Model file for the job. Use its own axes, mm. Face numbers are marked on the shaded views. Coordinates: 2 decimals unless noted, no trailing zeros. Order: outer loops, then holes, each group sorted by start corner. A loop starts at its lowest first (then second) coordinate and runs counter-clockwise, first axis right, second up.
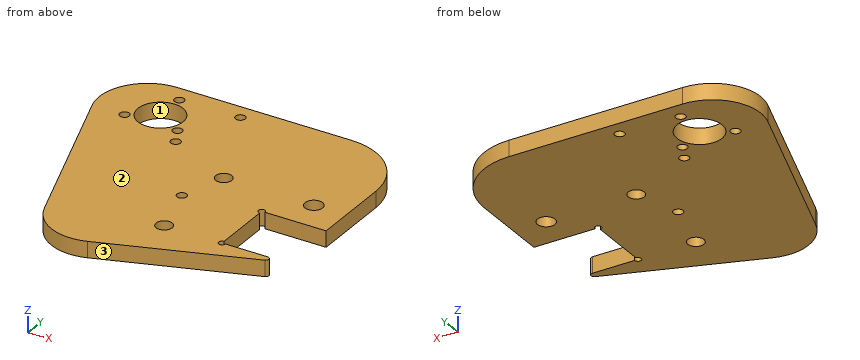
from build123d import *

# Parameters (mm, degrees)
SKETCH_1_R          = 7
SKETCH_1_R_2        = 1.5
SKETCH_1_R_3        = 2.5
EXTRUDE_1_DEPTH     = 5
FILLET_1_R          = 1
SKETCH_2_R          = 1.5
SKETCH_2_R_2        = 2.75
CUT_EXTRUDE_1_DEPTH = 10
SKETCH_3_R          = 1.5
CUT_EXTRUDE_2_DEPTH = 10
SKETCH_4_R          = 1.025
CUT_EXTRUDE_3_DEPTH = 30


with BuildPart() as part:
    # 草图1 → 凸台-拉伸1 (new body)
    with BuildSketch(Plane.XY):
        with BuildLine():
            Line((70, -30), (70, -5))
            ThreePointArc((70, -5), (64.142135624, 9.142135624), (50, 15))
            Line((50, 15), (-4.038673683, 15))
            ThreePointArc((-4.038673683, 15), (-16.237067712, 8.729214347), (-18.236326506, -4.840108917))
            Line((-18.236326506, -4.840108917), (0.10369211, -58.637496855))
            ThreePointArc((0.10369211, -58.637496855), (7.762372735, -67.297085809), (19.305024689, -67.938222033))
            Line((19.305024689, -67.938222033), (70, -50))
            Line((70, -50), (50, -50))
            Line((50, -50), (50, -30))
            Line((50, -30), (70, -30))
        make_face()
        Circle(SKETCH_1_R, mode=Mode.SUBTRACT)
        with Locations((0, 9.5)):
            Circle(SKETCH_1_R_2, mode=Mode.SUBTRACT)
        with Locations((8.227241336, -4.75)):
            Circle(SKETCH_1_R_2, mode=Mode.SUBTRACT)
        with Locations((-8.227241336, -4.75)):
            Circle(SKETCH_1_R_2, mode=Mode.SUBTRACT)
        with Locations((32, -50)):
            Circle(SKETCH_1_R_3, mode=Mode.SUBTRACT)
        with Locations((32, -20)):
            Circle(SKETCH_1_R_3, mode=Mode.SUBTRACT)
    extrude(amount=EXTRUDE_1_DEPTH)

    # 圆角1
    fillet_1_edges = [part.edges().sort_by_distance(p)[0] for p in [
        (70, -50, 2.5),
    ]]
    fillet(fillet_1_edges, radius=FILLET_1_R)

    # 草图2 → 切除-拉伸1 (cut)
    with BuildSketch(Plane.XY.offset(5)):
        with Locations((27.5, -33.82)):
            Circle(SKETCH_2_R)
        with Locations((18.66, 10)):
            Circle(SKETCH_2_R)
        with Locations((60, -20)):
            Circle(SKETCH_2_R_2)
    extrude(amount=-CUT_EXTRUDE_1_DEPTH, mode=Mode.SUBTRACT)

    # 草图3 → 切除-拉伸2 (cut)
    with BuildSketch(Plane.XY.offset(5)):
        with Locations((10.914424012, -10)):
            Circle(SKETCH_3_R)
    extrude(amount=-CUT_EXTRUDE_2_DEPTH, mode=Mode.SUBTRACT)

    # 草图4 → 切除-拉伸3 (cut, symmetric)
    with BuildSketch(Plane(origin=(0, 0, 0), x_dir=(-1, 0, 0), z_dir=(0, 0, -1))):
        with Locations((-50, -50)):
            Circle(SKETCH_4_R)
        with Locations((-50, -30)):
            Circle(SKETCH_4_R)
    extrude(amount=CUT_EXTRUDE_3_DEPTH, both=True, mode=Mode.SUBTRACT)


solid = part.part
Q1. Cut at A-A, the plane z = 1. Count the separate pieces of the cut face and the enclosed holes in it, plus the area to 3 significant figures.
Established:
separate pieces: 1
enclosed holes: 10
area: 5,390 mm2
Q2. Probe line 1 (Y direction, x = 1, z = 4); line 2 (X direction, y = -22, z = 0.4); line 3 (Y direction, x = 32, z = 1.95). List the from-to ranges inside material, lowest first.
Established:
line 1: y = -60.73 to -6.93, 6.93 to 8.38, 10.62 to 15
line 2: x = -12.39 to 30.5, 33.5 to 58.11, 61.89 to 70
line 3: y = -63.45 to -52.5, -47.5 to -22.5, -17.5 to 15
Q3. Cut at D-D, the plane y = -56. List the corners of the cut face in (x, z), plus the area to 3 significant figures.
Established:
outline: (-0.8, 0) - (53.04, 0) - (53.04, 5) - (-0.8, 5) - close
area: 269 mm2
Q4. Cut at C-C, the plane x = 5. List the corners of the cut face in (y, z), plus the area to 3 significant figures.
Established:
outline: (-65.57, 0) - (-4.9, 0) - (-4.9, 5) - (-65.57, 5) - close; (4.9, 0) - (15, 0) - (15, 5) - (4.9, 5) - close
area: 354 mm2
Q5. Mould opens along X. For the marked faces 1, 2 and 3 say: pulls with the +X half, pulls with the -X half, needs draft (parallel to the pull), parting line crosses it, or undercut.
Established:
face 1: undercut
face 2: needs draft
face 3: pulls with the +X half
Q6. Drop flat-ended pins along their axis: P1, Ø1.8, axis at x = 0, y = 9.5, coming from the +Z side; P2, Ø1, axis at y = -40, z = 3.5, coming from the -X side. Give the stop position or say it passes through.
Established:
P1: passes through
P2: stops at x = -6.42
Q7. Cut at B-B, the plane y = 0. List the corners of the cut face in (x, z), plus the area to 3 significant figures.
Established:
outline: (-19.04, 0) - (-7, 0) - (-7, 5) - (-19.04, 5) - close; (7, 0) - (69.36, 0) - (69.36, 5) - (7, 5) - close
area: 372 mm2
